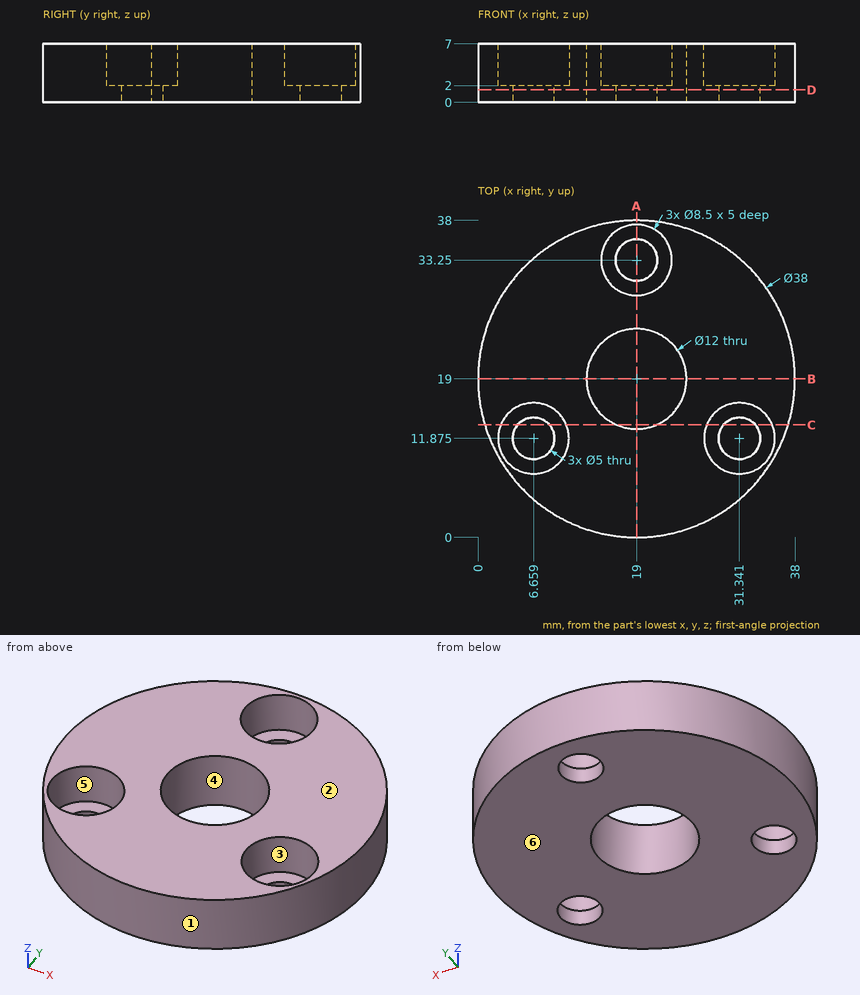
The drawing under review shows one solid part. Ordinate dimensions are in mm from its lowest x, y, z. A direction names the side the tool comes from. Coordinates: 2 decimals unless noted, no trailing zeros. Write each loop counter-clockwise with the first axis right and the second up, starting at its lowest first coordinate (ties: lowest second). Pieces come first, ordered by that corner, then holes. Notation, with made-up numbers: M -31,35.25 L 9,35.25 A6 ccw 9,46.25 Z; hole C 30.5,81.5 d6. An arc over 180 degrees is marked long. Put each result on its own line as item: value.
1) Add section B-B on y = 19. Give the boundary of the cut face in (x, z).
Computed:
outline: M 0,0 L 13,0 L 13,7 L 0,7 Z; M 25,0 L 38,0 L 38,7 L 25,7 Z
2) For the marked faces 5 and 6, list the 3-axis set-ups (+Z, -Z, +X, -X, +Y, -Y) from which the entire face can be reached by the end or side of a thin tool; tool diameter is ignored.
Computed:
face 5: +Z
face 6: -Z, +X, -X, +Y, -Y
3) Add section A-A on x = 19. Give the boundary of the cut face in (y, z).
Computed:
outline: M 0,0 L 13,0 L 13,7 L 0,7 Z; M 25,0 L 30.75,0 L 30.75,2 L 29,2 L 29,7 L 25,7 Z; M 35.75,0 L 38,0 L 38,7 L 37.5,7 L 37.5,2 L 35.75,2 Z
4) Add section C-C on y = 13.5. Give the boundary of the cut face in (x, z).
Computed:
outline: M 0.81,0 L 4.76,0 L 4.76,2 L 2.73,2 L 2.73,7 L 0.81,7 Z; M 8.56,0 L 16.6,0 L 16.6,7 L 10.59,7 L 10.59,2 L 8.56,2 Z; M 21.4,0 L 29.44,0 L 29.44,2 L 27.41,2 L 27.41,7 L 21.4,7 Z; M 33.24,0 L 37.19,0 L 37.19,7 L 35.27,7 L 35.27,2 L 33.24,2 Z
5) Wall thickness on probe 1 along Y at (x, z) = (19, 4); probe 2 along Y at (x, z) = (19, 1.1); probe 3 along X at (y, z) = (12, 1.25): over which ranges is each line inside the solid? List them lowest first. Write a range as [from, to].
Computed:
probe 1: y = [0, 13], [25, 29], [37.5, 38]
probe 2: y = [0, 13], [25, 30.75], [35.75, 38]
probe 3: x = [1.34, 4.16], [9.16, 28.84], [33.84, 36.66]
6) Draft analysis for pull direction Y (two halves, no side actions). For the marked faces 1, 2, 3 and 4, state which applies: released by +Y, released by -Y, zero draft, split by the parting line, or undercut.
Computed:
face 1: split by the parting line
face 2: zero draft
face 3: undercut
face 4: undercut
7) Add section D-D on z = 1.5. Give the boundary of the cut face in (x, y) (3 decimals).
Computed:
outline: C 19,19 d38; hole C 6.659,11.875 d5; hole C 19,19 d12; hole C 19,33.25 d5; hole C 31.341,11.875 d5
8) Clearance check with flat-ended pins moving along their axes: pin 1 Ø7 at (x, y) = (31.34, 11.88) entering from -Z; pin 2 Ø4 at (x, y) = (19, 31.5) entering from +Z; pin 3 Ø4.5 at (x, y) = (6.66, 11.88) entering from -Z. State where each tip first meets the part, or that it passes through.
Computed:
pin 1: stops at z = 0
pin 2: stops at z = 2
pin 3: passes through
